from build123d import *

# Parameters (mm, degrees)
F1_R     = 17.5
F1_R_2   = 13.5
F2_DEPTH = 15
F4_W     = 5
F4_H     = 3.8615576923
F5_DEPTH = 15
F6_COUNT = 4
F7_W     = 36.0574051738
F7_H     = 36.043446511
F7_R     = 13.5
F8_DEPTH = 10
F9_SIZE  = 10
F10_R    = 0.5
F11_R    = 0.5


with BuildPart() as f2:
    # F1 (on face) → F2 (new body)
    with BuildSketch(Plane.XY):
        Circle(F1_R)
        Circle(F1_R_2, mode=Mode.SUBTRACT)
    extrude(amount=F2_DEPTH)

    # F4 (on Top) → F5 (join)
    with BuildSketch(Plane.XY):
        with Locations((0, 12.4307788461)):
            Rectangle(F4_W, F4_H)
    extrude(amount=F5_DEPTH)

    # F6: F2 ×4 about axis
    f6_axis = Axis((0, 0, 0), (0, 0, 1))


with BuildPart() as f2_1:
    add(f2.part)
    for i in range(1, F6_COUNT):
        add(f2.part.rotate(f6_axis, i * 360 / F6_COUNT))

    # F7 (on face) → F8 (join)
    with BuildSketch(Plane.XY):
        Rectangle(F7_W, F7_H)
        Circle(F7_R, mode=Mode.SUBTRACT)
    extrude(amount=F8_DEPTH)

    # F9
    f9_edges = [f2_1.edges().sort_by_distance(p)[0] for p in [
        (18.028703, 18.021723, 5),
        (-18.028703, 18.021723, 5),
        (-18.028703, -18.021723, 5),
        (18.028703, -18.021723, 5),
    ]]
    chamfer(f9_edges, length=F9_SIZE)

    # F10
    f10_edges = [f2_1.edges().sort_by_distance(p)[0] for p in [
        (-17.5, 0, 10),
    ]]
    fillet(f10_edges, radius=F10_R)

    # F11
    f11_edges = [f2_1.edges().sort_by_distance(p)[0] for p in [
        (-17.5, 0, 15),
    ]]
    fillet(f11_edges, radius=F11_R)


solid = f2_1.part
Can you work these out from the model? Positions are in its coordinate system, mm. A direction names the side the tool comes from. Coordinates: 2 decimals unless noted, no trailing zeros. Loops run counter-clockwise (first coordinate to the right, second up) from the corner with the lowest first, then second, coordinate; pieces in that order, holes last. Notation, with made-up numbers: (-26, -5) - (31, -5) arc R35 cw to (31, 30) - close; hole circle Ø2 at (-36, -25.75). An arc over 180 degrees is marked (long way). Answer as a JSON object with one key per item and string values. Group by question number.
Item 1: If we mould it in two halves opening along Y, with no side actions, what happens to faces 1 (the face through (-13.887, -10.648, 12.472)), 2 (the face through (9.626, 9.466, 7.395)), 3 (the face through (0, 12, 0)), 4 (the face through (0, -18.022, 5))? For each: released by +Y, released by -Y, zero draft, split by the parting line, or undercut.
Item 2: On a 3-axis mill with a long thin cutter (end or side, diameter ignored), from which of +Z, -Z, +X, -X, +Y, -Y can I reach the whole of each face in a straight line? I mean faces 5 (the face through (-10.8, 14.8, 10)), 6 (the face through (-11, 0, 15)), 7 (the face through (10.5, 0, 7)). Say none if no direction works.
Item 3: If I drill on L1, parallel to X at y = -1.5, z = 4.5; L2, parallel to X at y = 11, z = 8; L3, parallel to Y at x = -12.5, z = 3.75, over which ranges is the centre line in solid material (lowest first)? Write a range as from..to.
Item 4: If we section it at A-A (z = 7.75): List the corners of the cut face in (x, y) for me.
Item 5: For pin 1 (2.5 mm diameter, centred on y = 1, z = 11, fed in from +X); pin 2 (3 mm diameter, centred on x = 12, z = 11, fed in from +Y); pin 3 (1.4 mm diameter, centred on x = -11.5, z = 4.5, fed in from -Y); pin 4 (0.8 mm diameter, centred on x = -11.5, z = 9.5, fed in from +Y), each with a flat end and sliding along its axis, tell me the tip position at first contact or that it passes through.
Returned:
{
 "1": {"face 1": "split by the parting line", "face 2": "undercut", "face 3": "zero draft", "face 4": "released by -Y"},
 "2": {"face 5": "+Z", "face 6": "+Z, +X, -X, +Y, -Y", "face 7": "+Z, -Z"},
 "3": {"L1": "x = -18.03..-10.5, 10.5..18.03", "L2": "x = -15.05..-7.83, -2.5..2.5, 7.83..15.05", "L3": "y = -13.55..-5.1, -2.5..2.5, 5.1..13.55"},
 "4": {"outline": "(-18.03, -8.02) - (-8.03, -18.02) - (8.03, -18.02) - (18.03, -8.02) - (18.03, 8.02) - (8.03, 18.02) - (-8.03, 18.02) - (-18.03, 8.02) - close; hole (-13.27, -2.5) arc R13.5 ccw to (-2.5, -13.27) - (-2.5, -10.5) - (2.5, -10.5) - (2.5, -13.27) arc R13.5 ccw to (13.27, -2.5) - (10.5, -2.5) - (10.5, 2.5) - (13.27, 2.5) arc R13.5 ccw to (2.5, 13.27) - (2.5, 10.5) - (-2.5, 10.5) - (-2.5, 13.27) arc R13.5 ccw to (-13.27, 2.5) - (-10.5, 2.5) - (-10.5, -2.5) - close"},
 "5": {"pin 1": "stops at x = 18.03", "pin 2": "stops at y = 15.17", "pin 3": "stops at y = -15.25", "pin 4": "stops at y = 14.95"}
}
